Autodesk Fusion 360 part; units mm, degrees
sketch "Esquisse1" plane through (0, 0, 0) normal (0, 1, 0) x (1, 0, 0)
  circle A0 centre (0, 0) radius 9
  circle A1 centre (0, 0) radius 7.5
  dimension "d1" = 18
  dimension "d6" = 15
extrude "Extrusion2" add sketch "Esquisse1" along normal blind 5 contours A0 | A1
extrude "Extrusion3" cut sketch "Esquisse1" along normal blind 3 contours A1
sketch "Esquisse2" plane through (0, 5, 0) normal (0, 1, 0) x (-1, 0, 0)
  circle A0 centre (0, 0) radius 9
  circle A1 centre (0, 0) radius 1
  dimension "d9" = 2
extrude "Extrusion4" cut sketch "Esquisse2" against normal blind 3 contours A1
CAD build for the part. Positions are in the model's coordinates, mm. A direction names the side the tool comes from. Round coordinates to 2 decimals unless told otherwise and drop trailing zeros. Order: outer loops, then holes, each group sorted by start corner. A loop starts at its lowest first (then second) coordinate and runs counter-clockwise, first axis right, second up. Notation, with made-up numbers: (78.25, 83) - (118.25, 83) arc R31 cw to (118.25, 119) - close; hole circle Ø8 at (47.5, 42.25). An arc over 180 degrees is marked (long way). Answer in a Markdown table with one row per item. Add a question column.
(1) Band-saw the part on A-A on x = 0. List the corners of the cut face in (y, z), and give its area (3 significant figures).
(2) 3-axis set-ups, long thin cutter, end or side, ignore diameter. For faces 4 (the face through (0, 3, 2)), 5 (the face through (-2, 0, -7.4)): which of +Z, -Z, +X, -X, +Y, -Y reach the whole face in a straight line?
(3) Band-saw the part on D-D on z = 4.5. List the corners of the cut face in (x, y).
(4) Drop flat-ended pins along their axis: pin 1 Ø5 at (x, z) = (3.5, -6.5) entering from -Y; pin 2 Ø1 at (x, y) = (1.5, 3) entering from -Z; pin 3 Ø3 at (x, z) = (0, 0) entering from -Y; pin 4 Ø3 at (y, z) = (3, -7) entering from +X. Give the stop position or say it passes through.
(5) Probe L1, parallel to X at y = 1.05, z = 0; L2, parallel to X at y = 1.65, z = 5. List the from-to ranges inside material, lowest first. Write a range as [from, to].
(6) Mould opens along Z. For faces 1 (the face through (-1.172, 2.465, 8.923)), 2 (the face through (-7.493, 1.479, 0.33)), 3 (the face through (0, 5, 2)) say: +Z half, -Z half, draft (parallel to the pull), parting line (faces both ways), or undercut.
(7) Band-saw the part on B-B on z = 0. List the corners of the cut face in (x, y), and give its area (3 significant figures).
(8) Band-saw the part on C-C on y = 1.9. List the corners of the cut face in (x, z), and give its area (3 significant figures).
Data:
| question | item | result |
|---|---|---|
| 1 | outline | (0, -9) - (5, -9) - (5, -1) - (3, -1) - (3, -7.5) - (0, -7.5) - close; (0, 7.5) - (3, 7.5) - (3, 1) - (5, 1) - (5, 9) - (0, 9) - close |
| 1 | area | 41.0 mm^2 |
| 2 | face 4 | -Y |
| 2 | face 5 | +Z, -Z, +X, -X, -Y |
| 3 | outline | (-7.79, 0) - (-6, 0) - (-6, 3) - (6, 3) - (6, 0) - (7.79, 0) - (7.79, 5) - (-7.79, 5) - close |
| 4 | pin 1 | stops at y = 0 |
| 4 | pin 2 | stops at z = -8.94 |
| 4 | pin 3 | stops at y = 3 |
| 4 | pin 4 | stops at x = 7.12 |
| 5 | L1 | x = [-9, -7.5], [7.5, 9] |
| 5 | L2 | x = [-7.48, -5.59], [5.59, 7.48] |
| 6 | face 1 | parting line |
| 6 | face 2 | undercut |
| 6 | face 3 | draft |
| 7 | outline | (-9, 0) - (-7.5, 0) - (-7.5, 3) - (-1, 3) - (-1, 5) - (-9, 5) - close; (1, 3) - (7.5, 3) - (7.5, 0) - (9, 0) - (9, 5) - (1, 5) - close |
| 7 | area | 41.0 mm^2 |
| 8 | outline | circle Ø18 at (0, 0); hole circle Ø15 at (0, 0) |
| 8 | area | 77.8 mm^2 |
